Answer from the drawing. Dimensions are ordinates in mm from the lowest x, y and z of the part. Round coordinates to 2 decimals unless told otherwise and drop trailing zeros. Loops run counter-clockwise (first coordinate to the right, second up) from the corner with the lowest first, then second, coordinate; pieces in that order, holes last. Notation, with made-up numbers: (44, -6.5) - (48, -6.5) arc R23 ccw to (48, 9.5) - close; hole circle Ø6 at (-21, -21.75). An arc over 180 degrees is marked (long way). Return JSON: item names as keys, results as strings.
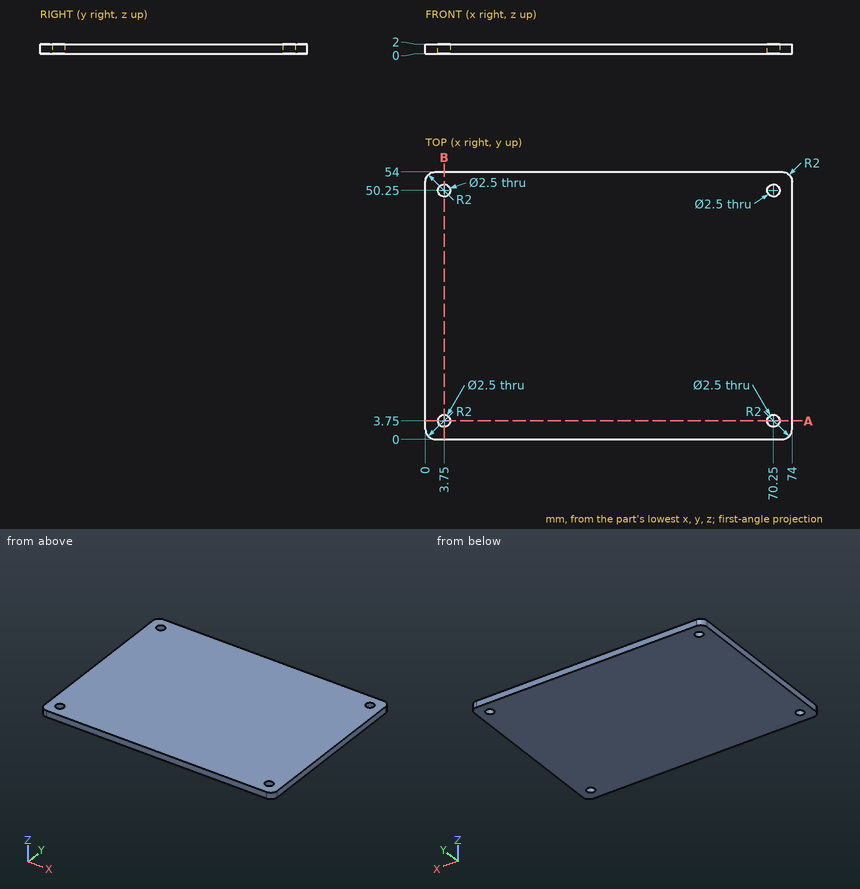
1) Section A-A (y = 3.75) is taken. Give the vertices of the cut face in (x, z), and give its area (3 significant figures).
Verdict:
{"outline": "(0, 0) - (2.5, 0) - (2.5, 2) - (0, 2) - close; (5, 0) - (69, 0) - (69, 2) - (5, 2) - close; (71.5, 0) - (74, 0) - (74, 2) - (71.5, 2) - close", "area": "138 mm2"}
2) Find the intervals of material crossed by L1, parallel to X at y = 50.25, z = 1.65; L2, parallel to Y at x = 70.25, z = 0.5, in increasing order.
Verdict:
{"L1": "x = 0 to 2.5, 5 to 69, 71.5 to 74", "L2": "y = 0 to 2.5, 5 to 49, 51.5 to 54"}
3) Section B-B (x = 3.75) is taken. Give the vertices of the cut face in (y, z), and give its area (3 significant figures).
Verdict:
{"outline": "(0, 0) - (2.5, 0) - (2.5, 2) - (0, 2) - close; (5, 0) - (49, 0) - (49, 2) - (5, 2) - close; (51.5, 0) - (54, 0) - (54, 2) - (51.5, 2) - close", "area": "98.0 mm2"}
